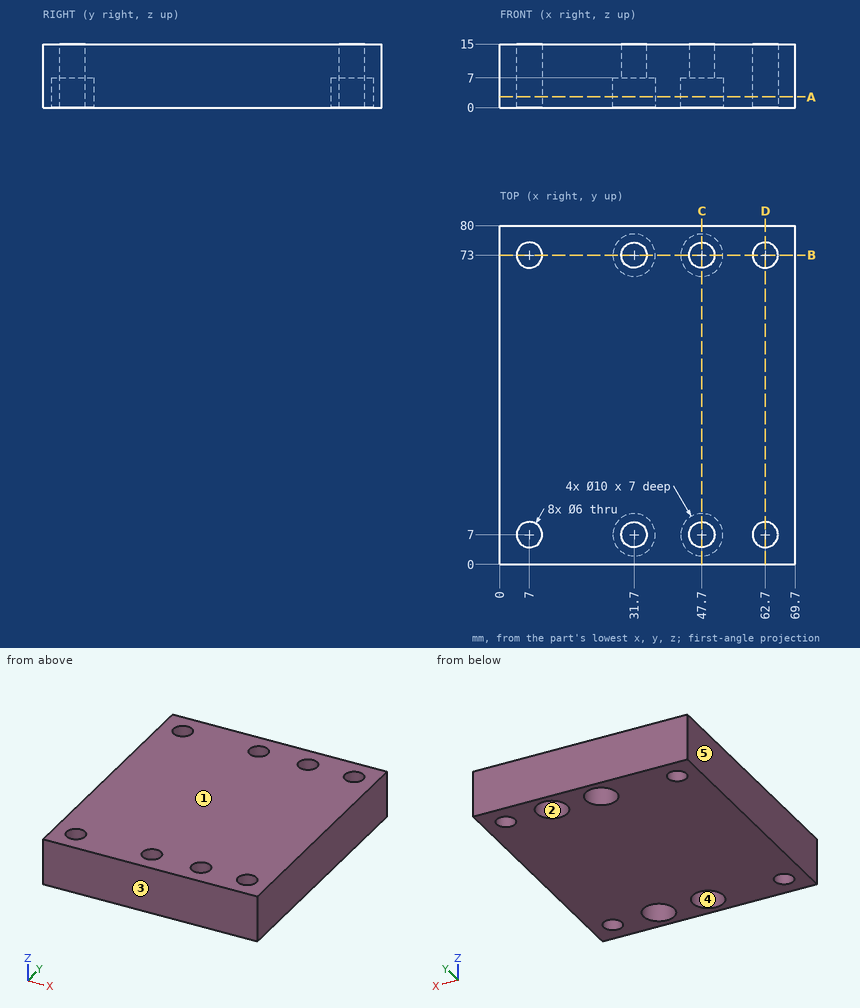
Job drawing, mm, ordinate dimensions from the low corner. One solid piece. A direction names the side the tool comes from. Coordinates: 2 decimals unless noted, no trailing zeros. Write each loop counter-clockwise with the first axis right and the second up, starting at its lowest first coordinate (ties: lowest second). Pieces come first, ordered by that corner, then holes. Notation, with made-up numbers: (29.5, 65) - (67.5, 65) arc R12 cw to (67.5, 83) - close; hole circle Ø3 at (-1, 14). An arc over 180 degrees is marked (long way). Use a Markdown table: item, result. Add a question column.
Item 1: Band-saw the part on B-B, the plane y = 73. Give the cut face in (x, z), and give its area (4 significant figures).
Item 2: Flat gauge pins, fed straight in: pin 1 (9.5 mm diameter, centred on x = 62.7, y = 73, fed in from -Z); pin 2 (5 mm diameter, centred on x = 29.5, y = 73, fed in from -Z). Where does each tip first touch, or does it go through?
Item 3: Band-saw the part on D-D, the plane x = 62.7. Give the cut face in (y, z).
Item 4: Drill centre lines: L1, parallel to Y at x = 47.7, z = 5.25; L2, parallel to Y at x = 62.7, z = 10. Where is each one in solid material? Low to high. Write a range as from..to.
Item 5: Mould opens along X. For the marked faces 3, 4 and 5 say: pulls with the +X half, pulls with the -X half, needs draft (parallel to the pull), parting line crosses it, or undercut.
Item 6: 3-axis set-ups, long thin cutter, end or side, ignore diameter. For the marked faces 1 and 2: which of +Z, -Z, +X, -X, +Y, -Y reach the whole face in a straight line?
Item 7: Band-saw the part on A-A, the plane z = 2.5. Give the number of separate pieces and of enclosed holes in the cut face, and give its area (3 significant figures).
Item 8: Band-saw the part on C-C, the plane x = 47.7. Give the cut face in (y, z).
Numbers:
| question | item | result |
|---|---|---|
| 1 | outline | (0, 0) - (4, 0) - (4, 15) - (0, 15) - close; (10, 0) - (26.7, 0) - (26.7, 7) - (28.7, 7) - (28.7, 15) - (10, 15) - close; (34.7, 7) - (36.7, 7) - (36.7, 0) - (42.7, 0) - (42.7, 7) - (44.7, 7) - (44.7, 15) - (34.7, 15) - close; (50.7, 7) - (52.7, 7) - (52.7, 0) - (59.7, 0) - (59.7, 15) - (50.7, 15) - close; (65.7, 0) - (69.7, 0) - (69.7, 15) - (65.7, 15) - close |
| 1 | area | 629.5 mm2 |
| 2 | pin 1 | z = 0 |
| 2 | pin 2 | z = 7 |
| 3 | outline | (0, 0) - (4, 0) - (4, 15) - (0, 15) - close; (10, 0) - (70, 0) - (70, 15) - (10, 15) - close; (76, 0) - (80, 0) - (80, 15) - (76, 15) - close |
| 4 | L1 | 0..2, 12..68, 78..80 |
| 4 | L2 | 0..4, 10..70, 76..80 |
| 5 | face 3 | needs draft |
| 5 | face 4 | undercut |
| 5 | face 5 | pulls with the -X half |
| 6 | face 1 | +Z, +X, -X, +Y, -Y |
| 6 | face 2 | -Z |
| 7 | separate pieces | 1 |
| 7 | enclosed holes | 8 |
| 7 | area | 5,150 mm2 |
| 8 | outline | (0, 0) - (2, 0) - (2, 7) - (4, 7) - (4, 15) - (0, 15) - close; (10, 7) - (12, 7) - (12, 0) - (68, 0) - (68, 7) - (70, 7) - (70, 15) - (10, 15) - close; (76, 7) - (78, 7) - (78, 0) - (80, 0) - (80, 15) - (76, 15) - close |
